Here's how the part is built. I have some questions about the finished solid (model axes, mm). A direction names the side the tool comes from. Round coordinates to 2 decimals unless told otherwise and drop trailing zeros. Write each loop counter-clockwise with the first axis right and the second up, starting at its lowest first coordinate (ties: lowest second). Pieces come first, ordered by that corner, then holes. Notation, with made-up numbers: (59, 66.5) - (64, 66.5) arc R27 ccw to (64, 97.5) - close; hole circle Ø1 at (39.5, 21.5). An arc over 180 degrees is marked (long way). One line per question, with ' | ' between items. Start each with the question number.
(1) For faces 1 (the flat face through (16.702, 1.972, 16.674)), 2 (the cylindrical face through (-20.8, 2, -21)), which set-ups out of +Z, -Z, +X, -X, +Y, -Y let a thin tool reach every point of the face, with its end or its side?
(2) Imagine slicing it at B-B (z = -14.5). Write out the boundary of the cut face in (x, y), plus the area to 3 significant figures.
(3) If I drill on L1, parallel to Z at x = 4.5, y = 2.5; L2, parallel to X at y = 1.6, z = 34.5; L3, parallel to X at y = 3.2, z = -15, over which ranges is the centre line in solid material (lowest first)?
(4) Imagine slicing it at C-C (x = -5). Write out the boundary of the cut face in (y, z), plus the area to 3 significant figures.
(5) Imagine slicing it at D-D (y = 1.2). Give the number of separate pieces and of enclosed holes in the cut face, plus the area to 3 significant figures.
(6) Will these pins go through, and if not, where does the flat tip stop? pin 1 (5 mm diameter, centred on x = 6, z = 24.5, fed in from +Y) (3 decimals); pin 2 (1.5 mm diameter, centred on x = 17.5, y = 2.5, fed in from -Z).
(7) Imagine slicing it at A-A (z = 5). Write out the boundary of the cut face in (x, y), plus the area to 3 significant figures.
from build123d import *

# Parameters (mm, degrees)
SKETCH_1_W          = 50
SKETCH_1_H          = 50
EXTRUDE_1_DEPTH     = 4
SKETCH_2_R          = 1.6
EXTRUDE_2_DEPTH     = 4
SKETCH_2_3_W        = 21
SKETCH_2_3_H        = 35
SKETCH_2_3_R        = 1.6
CUT_EXTRUDE_1_DEPTH = 4
FILLET_1_R          = 14
FILLET_2_R          = 14


with BuildPart() as part:
    # Sketch 1 → Extrude 1 (new body)
    with BuildSketch(Plane(origin=(0, 0, 0), x_dir=(1, 0, 0), z_dir=(0, 1, 0))):
        Rectangle(SKETCH_1_W, SKETCH_1_H)
        Polygon((15.708195736, 17.66756085), (17.667918398, 15.708099932), (20.344722661, 16.425539082), (21.061804264, 19.10243915), (19.102081602, 21.061900068), (16.425277339, 20.344460918), align=None, mode=Mode.SUBTRACT)
        Polygon((-17.66756085, 15.708195736), (-15.708099932, 17.667918398), (-16.425539082, 20.344722661), (-19.10243915, 21.061804264), (-21.061900068, 19.102081602), (-20.344460918, 16.425277339), align=None, mode=Mode.SUBTRACT)
        Polygon((17.66756085, -15.708195736), (15.708099932, -17.667918398), (16.425539082, -20.344722661), (19.10243915, -21.061804264), (21.061900068, -19.102081602), (20.344460918, -16.425277339), align=None, mode=Mode.SUBTRACT)
        Polygon((-15.708195736, -17.66756085), (-17.667918398, -15.708099932), (-20.344722661, -16.425539082), (-21.061804264, -19.10243915), (-19.102081602, -21.061900068), (-16.425277339, -20.344460918), align=None, mode=Mode.SUBTRACT)
    extrude(amount=EXTRUDE_1_DEPTH)

    # Sketch 2 → Extrude 2 (add)
    with BuildSketch(Plane.XZ):
        with BuildLine():
            ThreePointArc((25, 25), (0, 39.469136454), (-25, 25))
            Line((-25, 25), (-10.5, 25))
            Line((-10.5, 25), (-10.5, 31))
            Line((-10.5, 31), (10.5, 31))
            Line((10.5, 31), (10.5, 25))
            Line((10.5, 25), (25, 25))
        make_face()
        with Locations(Location((-5, 35.5, 0), (0, 0, 270))):
            Circle(SKETCH_2_R, mode=Mode.SUBTRACT)
        with Locations(Location((5, 35.5, 0), (0, 0, 270))):
            Circle(SKETCH_2_R, mode=Mode.SUBTRACT)
    extrude(amount=-EXTRUDE_2_DEPTH)

    # Sketch 2_3 → Cut-Extrude 1 (cut)
    with BuildSketch(Plane.XZ):
        with Locations((0, 7.5)):
            Rectangle(SKETCH_2_3_W, SKETCH_2_3_H)
        with Locations(Location((-5, -14.5, 0), (0, 0, 270))):
            Circle(SKETCH_2_3_R)
        with Locations(Location((5, -14.5, 0), (0, 0, 270))):
            Circle(SKETCH_2_3_R)
    extrude(amount=-CUT_EXTRUDE_1_DEPTH, mode=Mode.SUBTRACT)

    # Fillet 1
    fillet_1_edges = [part.edges().sort_by_distance(p)[0] for p in [
        (-25, 2, -25),
        (25, 2, -25),
    ]]
    fillet(fillet_1_edges, radius=FILLET_1_R)

    # Fillet 2
    fillet_2_edges = [part.edges().sort_by_distance(p)[0] for p in [
        (25, 2, 25),
        (-25, 2, 25),
    ]]
    fillet(fillet_2_edges, radius=FILLET_2_R)


solid = part.part
Check sheet entries:
1) face 1: +Y, -Y | face 2: -Z, -X, +Y, -Y
2) outline: (-24.56, 0) - (-6.6, 0) - (-6.6, 4) - (-24.56, 4) - close; (-3.4, 0) - (3.4, 0) - (3.4, 4) - (-3.4, 4) - close; (6.6, 0) - (24.56, 0) - (24.56, 4) - (6.6, 4) - close | area: 171 mm^2
3) L1: -25 to -16.02, -12.98 to -10, 31 to 33.98, 37.02 to 39.12 | L2: -16.18 to -6.25, -3.75 to 3.75, 6.25 to 16.18 | L3: -24.42 to -6.52, -3.48 to 3.48, 6.52 to 24.42
4) outline: (0, -25) - (4, -25) - (4, -16.1) - (0, -16.1) - close; (0, -12.9) - (4, -12.9) - (4, -10) - (0, -10) - close; (0, 31) - (4, 31) - (4, 33.9) - (0, 33.9) - close; (0, 37.1) - (4, 37.1) - (4, 39.03) - (0, 39.03) - close | area: 66.5 mm^2
5) separate pieces: 1 | enclosed holes: 9 | area: 1,950 mm^2
6) pin 1: through | pin 2: z = -23.76
7) outline: (-25, 0) - (-10.5, 0) - (-10.5, 4) - (-25, 4) - close; (10.5, 0) - (25, 0) - (25, 4) - (10.5, 4) - close | area: 116 mm^2
